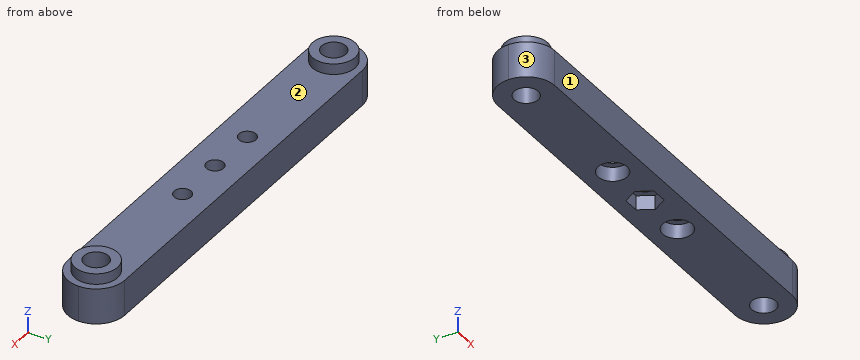
```python
from build123d import *

# Parameters (mm, degrees)
F2_W      = 61
F2_H      = 8
F2_R      = 3
F5_DEPTH  = 5
F1_R      = 3
F1_R_2    = 1.7
F6_DEPTH  = 6.5
F0_R      = 1.7
F7_DEPTH  = 12.5
F3_R      = 2.05
F8_DEPTH  = 2
F9_DEPTH  = 2
F10_R     = 3.99999
F4_R      = 1.2
F11_DEPTH = 6.501


# Not quite as in the source:
# - a fillet or chamfer is up to 0.001 mm smaller than in the source, because OpenCascade refuses the exact size


with BuildPart() as f5:
    # F2 (on face) → F5 (new body)
    with BuildSketch(Plane.XY):
        with Locations((0, 38)):
            Rectangle(F2_W, F2_H)
        with Locations((-26.5, 38)):
            Circle(F2_R, mode=Mode.SUBTRACT)
        Polygon((1.1402667816, 36.025), (0, 36.025), (-1.1402667816, 36.025), (-2.2805335633, 38), (-1.1402667816, 39.975), (0, 39.975), (1.1402667816, 39.975), (2.2805335633, 38), align=None, mode=Mode.SUBTRACT)
        with Locations((26.5, 38)):
            Circle(F2_R, mode=Mode.SUBTRACT)
        Polygon((-1.1402667816, 36.025), (0, 36.025), (1.1402667816, 36.025), (2.2805335633, 38), (1.1402667816, 39.975), (0, 39.975), (-1.1402667816, 39.975), (-2.2805335633, 38), align=None)
        with Locations((-26.5, 38)):
            Circle(F2_R)
        with Locations((26.5, 38)):
            Circle(F2_R)
    extrude(amount=F5_DEPTH)

    # F1 (on Top) → F6 (join)
    with BuildSketch(Plane.XY):
        with Locations((-26.5, 38)):
            Circle(F1_R)
        with Locations((-26.5, 38)):
            Circle(F1_R_2, mode=Mode.SUBTRACT)
        with Locations((26.5, 38)):
            Circle(F1_R)
        with Locations((26.5, 38)):
            Circle(F1_R_2, mode=Mode.SUBTRACT)
    extrude(amount=F6_DEPTH)

    # F0 (on Top) → F7 (cut, symmetric)
    with BuildSketch(Plane.XY):
        with Locations((-26.5, 38)):
            Circle(F0_R)
        with Locations((26.5, 38)):
            Circle(F0_R)
        with Locations((-26.5, -38)):
            Circle(F0_R)
        with Locations((26.5, -38)):
            Circle(F0_R)
    extrude(amount=F7_DEPTH, both=True, mode=Mode.SUBTRACT)

    # F3 (on face) → F8 (cut)
    with BuildSketch(Plane.XY):
        with Locations((-7.225, 38)):
            Circle(F3_R)
        with Locations((7.225, 38)):
            Circle(F3_R)
    extrude(amount=F8_DEPTH, mode=Mode.SUBTRACT)

    # F2 (on face) → F9 (cut)
    with BuildSketch(Plane.XY):
        Polygon((-1.1402667816, 36.025), (0, 36.025), (1.1402667816, 36.025), (2.2805335633, 38), (1.1402667816, 39.975), (0, 39.975), (-1.1402667816, 39.975), (-2.2805335633, 38), align=None)
    extrude(amount=F9_DEPTH, mode=Mode.SUBTRACT)

    # F10 (radius 4 in the source; OpenCascade refuses exactly that, so slightly less here)
    f10_edges = [f5.edges().sort_by_distance(p)[0] for p in [
        (-30.5, 42, 2.5),
        (-30.5, 34, 2.5),
        (30.5, 42, 2.5),
        (30.5, 34, 2.5),
    ]]
    fillet(f10_edges, radius=F10_R)

    # F4 (on face) → F11 (cut, through all)
    with BuildSketch(Plane.XY):
        with Locations((-7.225, 38)):
            Circle(F4_R)
        with Locations((0, 38)):
            Circle(F4_R)
        with Locations((7.225, 38)):
            Circle(F4_R)
    extrude(amount=F11_DEPTH, mode=Mode.SUBTRACT)


solid = f5.part
```
Work out the finished part from the listing and answer in its coordinate system (mm). Face numbers are marked on the shaded views. Round coordinates to 2 decimals unless told otherwise and drop trailing zeros. Write each loop counter-clockwise with the first axis right and the second up, starting at its lowest first coordinate (ties: lowest second). Pieces come first, ordered by that corner, then holes.
1) A cutting plane is placed at A-A on x = 0. Determine the outline of the cut face in (y, z) (3 decimals), and give its area (3 significant figures).
2) A cutting plane is placed at C-C on x = 19.5. Determine the outline of the cut face in (y, z), and give its area (3 significant figures).
3) A cutting plane is placed at B-B on z = 3.25. Give the number of separate pieces and of enclosed holes in the cut face, and give its area (3 significant figures).
4) Consider probe 1 along X at (y, z) = (39.75, 1.75); probe 2 along X at (y, z) = (39, 4.5); probe 3 along Y at (x, z) = (0, 2.6). Determine where each line is inside the solid, lowest interval first.
5) Determine the mould class of the marked faces 1, 2 and 3 for opening direction X: pulls with the +X half, pulls with the -X half, needs draft (parallel to the pull), parting line crosses it, or undercut.
6) Flat-ended cylindrical pins translate along their axes: P1, Ø1, axis at x = -2.5, y = 40, coming from the +Z side; P2, Ø4.5, axis at x = -8, y = 37.5, coming from the -Z side; P3, Ø2.5, axis at x = -7.225, y = 38, coming from the -Z side. Find the tip coordinate at first contact, or state that the pin passes through.
Entries:
1. outline: (34, 0) - (36.025, 0) - (36.025, 2) - (36.8, 2) - (36.8, 5) - (34, 5) - close; (39.2, 2) - (39.975, 2) - (39.975, 0) - (42, 0) - (42, 5) - (39.2, 5) - close
1. area: 24.9 mm2
2. outline: (34, 0) - (42, 0) - (42, 5) - (34, 5) - close
2. area: 40.0 mm2
3. separate pieces: 1
3. enclosed holes: 5
3. area: 443 mm2
4. probe 1: x = -30.1 to -8.29, -6.16 to -1.27, 1.27 to 6.16, 8.29 to 30.1
4. probe 2: x = -30.37 to -27.87, -25.13 to -7.89, -6.56 to -0.66, 0.66 to 6.56, 7.89 to 25.13, 27.87 to 30.37
4. probe 3: y = 34 to 36.8, 39.2 to 42
5. face 1: needs draft
5. face 2: undercut
5. face 3: pulls with the -X half
6. P1: stops at z = 5
6. P2: stops at z = 0
6. P3: stops at z = 2
